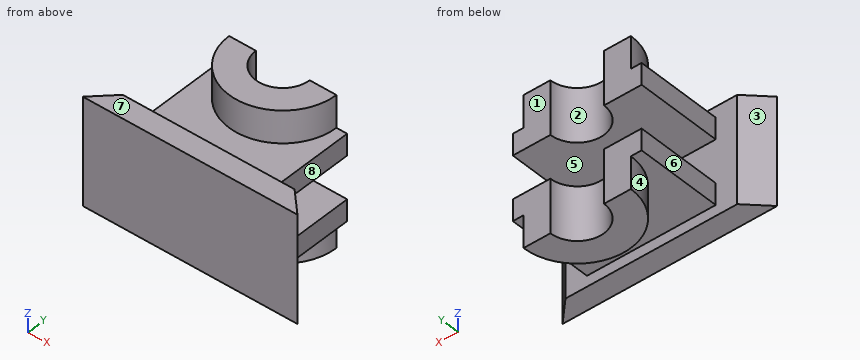
```python
from build123d import *

# Parameters (mm, degrees)
BOSS_EXTRUDE1_DEPTH = 25
BOSS_EXTRUDE2_START = 10
BOSS_EXTRUDE2_DEPTH = 10
BOSS_EXTRUDE3_START = -20
BOSS_EXTRUDE3_DEPTH = 10
BOSS_EXTRUDE4_START = -35
BOSS_EXTRUDE4_DEPTH = 25
BOSS_EXTRUDE5_START = 10
BOSS_EXTRUDE5_DEPTH = 25


with BuildPart() as part:
    # Sketch1 → Boss-Extrude1 (new, symmetric)
    with BuildSketch(Plane.XY):
        Polygon((50, 10), (50, 0), (100, 0), (90, 10), (80, 10), align=None)
        Polygon((10, 10), (0, 0), (50, 0), (50, 10), (20, 10), align=None)
    extrude(amount=BOSS_EXTRUDE1_DEPTH, both=True)

    # Sketch1<3> → Boss-Extrude2 (add)
    with BuildSketch(Plane.XY.offset(BOSS_EXTRUDE2_START)):
        with BuildLine():
            Line((50, 25), (50, 10))
            Line((50, 10), (80, 10))
            Line((80, 10), (80, 50))
            Line((80, 50), (75, 50))
            ThreePointArc((75, 50), (67.67766953, 32.32233047), (50, 25))
        make_face()
        with BuildLine():
            Line((20, 10), (50, 10))
            Line((50, 10), (50, 25))
            ThreePointArc((50, 25), (32.32233047, 32.32233047), (25, 50))
            Line((25, 50), (20, 50))
            Line((20, 50), (20, 10))
        make_face()
    extrude(amount=BOSS_EXTRUDE2_DEPTH)

    # Sketch1<4> → Boss-Extrude3 (add)
    with BuildSketch(Plane.XY.offset(BOSS_EXTRUDE3_START)):
        with BuildLine():
            Line((50, 25), (50, 10))
            Line((50, 10), (80, 10))
            Line((80, 10), (80, 50))
            Line((80, 50), (75, 50))
            ThreePointArc((75, 50), (67.67766953, 32.32233047), (50, 25))
        make_face()
        with BuildLine():
            Line((20, 10), (50, 10))
            Line((50, 10), (50, 25))
            ThreePointArc((50, 25), (32.32233047, 32.32233047), (25, 50))
            Line((25, 50), (20, 50))
            Line((20, 50), (20, 10))
        make_face()
    extrude(amount=BOSS_EXTRUDE3_DEPTH)

    # Sketch1<5> → Boss-Extrude4 (add)
    with BuildSketch(Plane.XY.offset(BOSS_EXTRUDE4_START)):
        with BuildLine():
            Line((37.5, 50), (25, 50))
            ThreePointArc((25, 50), (50, 25), (75, 50))
            Line((75, 50), (62.5, 50))
            ThreePointArc((62.5, 50), (50, 37.5), (37.5, 50))
        make_face()
    extrude(amount=BOSS_EXTRUDE4_DEPTH)

    # Sketch1<6> → Boss-Extrude5 (add)
    with BuildSketch(Plane.XY.offset(BOSS_EXTRUDE5_START)):
        with BuildLine():
            Line((37.5, 50), (25, 50))
            ThreePointArc((25, 50), (50, 25), (75, 50))
            Line((75, 50), (62.5, 50))
            ThreePointArc((62.5, 50), (50, 37.5), (37.5, 50))
        make_face()
    extrude(amount=BOSS_EXTRUDE5_DEPTH)


solid = part.part
```
The listing builds one solid part. Answer for the finished solid, in the listing's coordinates (mm). Face numbers are marked on the shaded views. A direction names the side the tool comes from. Give positions to 0.01 mm unless a question says otherwise; leave off trailing zeros. Order: outer loops, then holes, each group sorted by start corner. A loop starts at its lowest first (then second) coordinate and runs counter-clockwise, first axis right, second up. Notation, with made-up numbers: (-33, -13) -> (2, -13) arc R16 cw to (2, 11) -> close; hole circle Ø6 at (-22.75, 49.25). An arc over 180 degrees is marked (long way). Answer as a JSON object with one key per item and string values. Group by question number.
Item 1: The part is cut by section D-D on x = 34. Write down the section's boundary in (y, z), and give its area (3 significant figures).
Item 2: The part is cut by section A-A on y = 29.5. Write down the section's boundary in (x, z).
Item 3: Determine the mould class of the marked faces 1, 2 and 3 for opening direction X: pulls with the +X half, pulls with the -X half, needs draft (parallel to the pull), parting line crosses it, or undercut.
Item 4: A tool of negligible diameter and unlimited length cuts with its end or side. For the marked faces 4, 5, 6, 7 and 8, from which of +Z, -Z, +X, -X, +Y, -Y can it reach the whole face along a straight path? Write none if from no direction.
Item 5: Consider L1, parallel to Z at x = 64, y = 32; L2, parallel to Z at x = 52.5, y = 17; L3, parallel to Y at x = 19, z = -24. Determine where each line is inside the solid, lowest interval first. Write a range as from..to.
Item 6: The part is cut by section B-B on x = 50. Write down the section's boundary in (y, z).
Item 7: Flat-ended cylindrical pins translate along their axes: pin 1 (15 mm diameter, centred on x = 68, z = -6, fed in from +Y); pin 2 (8 mm diameter, centred on y = 20.5, z = 16, fed in from -X); pin 3 (10 mm diameter, centred on y = 11.5, z = -9, fed in from +X); pin 4 (3 mm diameter, centred on y = 39.5, z = 15.5, fed in from +X). Find the tip coordinate at first contact, or state that the pin passes through.
Item 8: The part is cut by section C-C on z = -5. Write down the section's boundary in (x, y).
Result set:
{
 "1": {"outline": "(0, -25) -> (10, -25) -> (10, -20) -> (30.79, -20) -> (30.79, -35) -> (50, -35) -> (50, -10) -> (10, -10) -> (10, 10) -> (50, 10) -> (50, 35) -> (30.79, 35) -> (30.79, 20) -> (10, 20) -> (10, 25) -> (0, 25) -> close", "area": "1,880 mm²"},
 "2": {"outline": "(20, -20) -> (35.69, -20) -> (35.69, -35) -> (64.31, -35) -> (64.31, -20) -> (80, -20) -> (80, -10) -> (20, -10) -> close; (20, 10) -> (80, 10) -> (80, 20) -> (64.31, 20) -> (64.31, 35) -> (35.69, 35) -> (35.69, 20) -> (20, 20) -> close"},
 "3": {"face 1": "needs draft", "face 2": "undercut", "face 3": "pulls with the -X half"},
 "4": {"face 4": "-Z", "face 5": "+X, -X, +Y", "face 6": "+Z, -Z, -X, +Y", "face 7": "+Z, +X, -X, -Y", "face 8": "+Z, -Z, +X, +Y"},
 "5": {"L1": "-35..-10, 10..35", "L2": "-20..-10, 10..20", "L3": "0..10"},
 "6": {"outline": "(0, -25) -> (10, -25) -> (10, -20) -> (25, -20) -> (25, -35) -> (37.5, -35) -> (37.5, -10) -> (10, -10) -> (10, 10) -> (37.5, 10) -> (37.5, 35) -> (25, 35) -> (25, 20) -> (10, 20) -> (10, 25) -> (0, 25) -> close"},
 "7": {"pin 1": "y = 50", "pin 2": "x = 20", "pin 3": "x = 93.5", "pin 4": "x = 80"},
 "8": {"outline": "(0, 0) -> (100, 0) -> (90, 10) -> (10, 10) -> close"}
}
